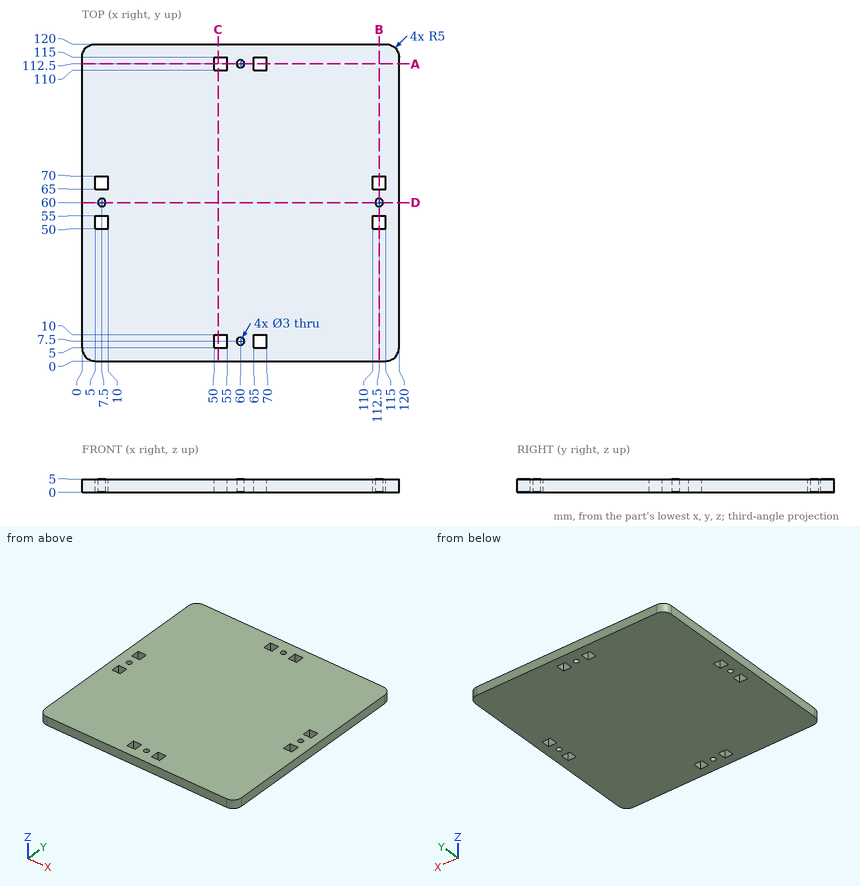
The figure shows three views and two pictorial views of one solid part (mm, origin at its lowest corner). Answer the questions. Round coordinates to 2 decimals unless told otherwise and drop trailing zeros. Write each loop counter-clockwise with the first axis right and the second up, starting at its lowest first coordinate (ties: lowest second). Pieces come first, ordered by that corner, then holes. Notation, with made-up numbers: (5.25, 86.5) - (51.25, 86.5) arc R20 cw to (51.25, 107.5) - close; hole circle Ø8 at (46.25, 27). An arc over 180 degrees is marked (long way). One line per question, with ' | ' between items. Start each with the question number.
1. This flat-tipped pin is pushed along its axis until it touches: pin 1 (2 mm diameter, centred on y = 42.5, z = 2.5, fed in from -X). Where does it stop, or does it pass through?
2. Section A-A (y = 112.5) is taken. Determine the outline of the cut face in (x, z).
3. Find the intervals of material crossed by probe 1 along Y at (x, z) = (60, 3.9); probe 2 along X at (y, z) = (7.5, 3.75); probe 3 along Y at (x, z) = (65.5, 3.95), in increasing order. Write a range as [from, to].
4. Section D-D (y = 60) is taken. Determine the outline of the cut face in (x, z).
5. Section C-C (x = 51.5) is taken. Determine the outline of the cut face in (y, z), and give its area (3 significant figures).
Filled in:
1) pin 1: x = 0
2) outline: (0, 0) - (50, 0) - (50, 5) - (0, 5) - close; (55, 0) - (58.5, 0) - (58.5, 5) - (55, 5) - close; (61.5, 0) - (65, 0) - (65, 5) - (61.5, 5) - close; (70, 0) - (120, 0) - (120, 5) - (70, 5) - close
3) probe 1: [0, 6], [9, 111], [114, 120] | probe 2: [0, 50], [55, 58.5], [61.5, 65], [70, 120] | probe 3: [0, 5], [10, 110], [115, 120]
4) outline: (0, 0) - (6, 0) - (6, 5) - (0, 5) - close; (9, 0) - (111, 0) - (111, 5) - (9, 5) - close; (114, 0) - (120, 0) - (120, 5) - (114, 5) - close
5) outline: (0, 0) - (5, 0) - (5, 5) - (0, 5) - close; (10, 0) - (110, 0) - (110, 5) - (10, 5) - close; (115, 0) - (120, 0) - (120, 5) - (115, 5) - close | area: 550 mm²
